For this review, take the finished solid that the model builds, in its own axes (mm). A direction names the side the tool comes from. Round coordinates to 2 decimals unless told otherwise and drop trailing zeros. Order: outer loops, then holes, each group sorted by start corner. A loop starts at its lowest first (then second) coordinate and runs counter-clockwise, first axis right, second up. Notation, with made-up numbers: M 41,51 L 55,51 A11 cw 55,71 Z; hole C -35.5,9.5 d3. An arc over 180 degrees is marked long. Use a Markdown table: item, result.
from build123d import *

# Parameters (mm, degrees)
SKETCH2_W           = 10
SKETCH2_H           = 3
BOSS_EXTRUDE1_DEPTH = 10
FILLET1_R           = 2
SKETCH3_R           = 1.6
CUT_EXTRUDE1_DEPTH  = 20.339079606
CUT_EXTRUDE2_DEPTH  = 1


with BuildPart() as part:
    # Sketch2 → Boss-Extrude1 (new body)
    with BuildSketch(Plane.XY):
        with Locations((-10, -1.5)):
            Rectangle(SKETCH2_W, SKETCH2_H)
        with BuildLine():
            Line((-7, 0), (-5, 0))
            ThreePointArc((-5, 0), (0, 5), (5, 0))
            Line((5, 0), (7, 0))
            ThreePointArc((7, 0), (0, 7), (-7, 0))
        make_face()
        with Locations((10, -1.5)):
            Rectangle(SKETCH2_W, SKETCH2_H)
    extrude(amount=BOSS_EXTRUDE1_DEPTH)

    # Fillet1
    fillet1_edges = [part.edges().sort_by_distance(p)[0] for p in [
        (-7, 0, 5),
        (7, 0, 5),
    ]]
    fillet(fillet1_edges, radius=FILLET1_R)

    # Sketch3 → Cut-Extrude1 (cut, through all)
    with BuildSketch(Plane(origin=(0, 0, 0), x_dir=(1, 0, 0), z_dir=(0, 1, 0))):
        with Locations(Location((11.8, -5, 0), (0, 0, 180))):
            Circle(SKETCH3_R)
        with Locations(Location((-11.8, -5, 0), (0, 0, 180))):
            Circle(SKETCH3_R)
    extrude(amount=-CUT_EXTRUDE1_DEPTH, mode=Mode.SUBTRACT)

    # Sketch4 → Cut-Extrude2 (cut)
    with BuildSketch(Plane(origin=(0, 0, 0), x_dir=(1, 0, 0), z_dir=(0, 1, 0))):
        Polygon((10.789637029, -6.75), (12.810362971, -6.75), (13.820725942, -5), (12.810362971, -3.25), (10.789637029, -3.25), (9.779274058, -5), align=None)
        Polygon((-12.810362971, -6.75), (-10.789637029, -6.75), (-9.779274058, -5), (-10.789637029, -3.25), (-12.810362971, -3.25), (-13.820725942, -5), align=None)
    extrude(amount=-CUT_EXTRUDE2_DEPTH, mode=Mode.SUBTRACT)


solid = part.part
Q1. Add section A-A (x = 11.8). Write out the cut boundary in (y, z).
Determined:
| item | result |
|---|---|
| outline | M -3,0 L 0,0 L 0,3.25 L -1,3.25 L -1,3.4 L -3,3.4 Z; M -3,6.6 L -1,6.6 L -1,6.75 L 0,6.75 L 0,10 L -3,10 Z |
Q2. Draft analysis for pull direction Z (two halves, no side actions). For faces 1 (the flat face through (-2, 5, 10)), 2 (the flat face through (10.3, -0.5, 5.9)), 3 (the flat face through (-2, 5, 0)), 4 (the flat face through (-10, -3, 5)), state which applies: pulls with the +Z half, pulls with the -Z half, needs draft (parallel to the pull), parting line crosses it, or undercut.
Determined:
| item | result |
|---|---|
| face 1 | pulls with the +Z half |
| face 2 | undercut |
| face 3 | pulls with the -Z half |
| face 4 | needs draft |
Q3. Clearance check with flat-ended pins moving along their axes: pin 1 (3 mm diameter, centred on y = 3, z = 3.5, fed in from +X); pin 2 (1.9 mm diameter, centred on x = -11.5, z = 5, fed in from +Y); pin 3 (1.9 mm diameter, centred on x = 11, z = 4.5, fed in from +Y); pin 4 (1.5 mm diameter, centred on x = -1, z = 4.5, fed in from -Y). State where each tip first meets the part, or that it passes through.
Determined:
| item | result |
|---|---|
| pin 1 | stops at x = 6.84 |
| pin 2 | passes through |
| pin 3 | stops at y = 0 |
| pin 4 | stops at y = 4.68 |
Q4. Machinability: for faces 5 (the flat face through (10, -3, 5)), 6 (the flat face through (-10, -1, 5)), 7 (the flat face through (-13.314, 0, 3.819)), which of the approach directions +Z, -Z, +X, -X, +Y, -Y give a long, thin tool a straight path to every point of the face, cutting with its end or side? Answer none if there is none.
Determined:
| item | result |
|---|---|
| face 5 | +Z, -Z, +X, -X, -Y |
| face 6 | +Y |
| face 7 | +Z, -Z, -X, +Y |
Q5. Add section B-B (z = 4). Write out the cut boundary in (x, y).
Determined:
| item | result |
|---|---|
| outline | M -15,-3 L -13.05,-3 L -13.05,-1 L -13.24,-1 L -13.24,0 L -15,0 Z; M -10.55,-3 L -5,-3 L -5,0 A5 cw 5,0 L 5,-3 L 10.55,-3 L 10.55,-1 L 10.36,-1 L 10.36,0 L 8.77,0 A2 cw 6.82,1.56 A7 ccw -6.82,1.56 A2 cw -8.77,0 L -10.36,0 L -10.36,-1 L -10.55,-1 Z; M 13.05,-3 L 15,-3 L 15,0 L 13.24,0 L 13.24,-1 L 13.05,-1 Z |
Q6. Wall thickness on line 1 along Z through (x, y) = (-11.8, -2.3); line 2 along X through (y, z) = (-1.25, 7.5); line 3 along X through (y, z) = (1.75, 1.75): over which ranges is each line inside the solid? List them lowest first. Write a range as [from, to].
Determined:
| item | result |
|---|---|
| line 1 | z = [0, 3.4], [6.6, 10] |
| line 2 | x = [-15, -5], [5, 15] |
| line 3 | x = [-6.78, -4.68], [4.68, 6.78] |
Q7. Add section D-D (x = 0). Write out the cut boundary in (y, z).
Determined:
| item | result |
|---|---|
| outline | M 5,0 L 7,0 L 7,10 L 5,10 Z |
Q8. Add section C-C (y = 4.5). Write out the cut boundary in (x, z).
Determined:
| item | result |
|---|---|
| outline | M -5.36,0 L -2.18,0 L -2.18,10 L -5.36,10 Z; M 2.18,0 L 5.36,0 L 5.36,10 L 2.18,10 Z |
